Here's how the part is built. I have some questions about the finished solid (model axes, mm). Face numbers are marked on the shaded views. A direction names the side the tool comes from. Coordinates: 2 decimals unless noted, no trailing zeros. Write each loop counter-clockwise with the first axis right and the second up, starting at its lowest first coordinate (ties: lowest second). Pieces come first, ordered by that corner, then holes.
Item 1: I want a section at A-A (y = 17). Please give me the cut outline in (x, z), and give its area (3 significant figures).
Item 2: I'm going to push flat-ended pins straight in: P1, Ø2.5, axis at x = 20, z = 0, coming from the +Y side; P2, Ø3.5, axis at x = 0, z = 20, coming from the +Y side; P3, Ø1.5, axis at y = 6.5, z = 4.5, coming from the -X side; P4, Ø10, axis at x = 20, z = -7.5, coming from the -Y side. Where does each tip first touch, or does it pass through?
Item 3: Please list where these lines run through material, in increasing order: line 1 (X direction, y = 18.1, z = 0); line 2 (Z direction, x = 1, y = 17); line 3 (Z direction, x = 2, y = 3).
Item 4: For the marked faces 4, 5 and 6, which set-ups out of +Z, -Z, +X, -X, +Y, -Y let a thin tool reach every point of the face, with its end or its side?
Item 5: If we mould it in two halves opening along Z, with no side actions, what happens to the marked faces 1, 2 and 3? For each: pulls with the +Z half, pulls with the -Z half, needs draft (parallel to the pull), parting line crosses it, or undercut.
Item 6: I want a section at C-C (z = 20). Please give me the cut outline in (x, y).
Item 7: I want a section at D-D (y = 11). Please give me the cut outline in (x, z).
Item 8: I want a section at B-B (x = 20). Please give me the cut outline in (y, z).
from build123d import *

# Parameters (mm, degrees)
SKETCH1_R           = 17.5
BOSS_EXTRUDE1_DEPTH = 16
SKETCH2_R           = 25
SKETCH2_R_2         = 12.5
BOSS_EXTRUDE2_DEPTH = 4
SKETCH3_R           = 1.5
CUT_EXTRUDE1_DEPTH  = 41.620192023
CHAMFER1_SIZE       = 1
SKETCH4_R           = 12.5
BOSS_EXTRUDE3_DEPTH = 4


with BuildPart() as part:
    # Sketch1 → Boss-Extrude1 (new body)
    with BuildSketch(Plane(origin=(0, 0, 0), x_dir=(1, 0, 0), z_dir=(0, 1, 0))):
        with Locations(Location((0, 0, 0), (0, 0, 270))):
            Circle(SKETCH1_R)
        Polygon((5.773502692, -10), (11.547005384, 0), (5.773502692, 10), (-5.773502692, 10), (-11.547005384, 0), (-5.773502692, -10), align=None, mode=Mode.SUBTRACT)
    extrude(amount=BOSS_EXTRUDE1_DEPTH)

    # Sketch2 → Boss-Extrude2 (add)
    with BuildSketch(Plane(origin=(0, 16, 0), x_dir=(1, 0, 0), z_dir=(0, 1, 0))):
        with Locations(Location((0, 0, 0), (0, 0, 270))):
            Circle(SKETCH2_R)
        with Locations(Location((0, 0, 0), (0, 0, 270))):
            Circle(SKETCH2_R_2, mode=Mode.SUBTRACT)
    extrude(amount=BOSS_EXTRUDE2_DEPTH)

    # Sketch3 → Cut-Extrude1 (cut, through all)
    with BuildSketch(Plane(origin=(0, 20, 0), x_dir=(1, 0, 0), z_dir=(0, 1, 0))):
        with Locations(Location((0, 20, 0), (0, 0, 270))):
            Circle(SKETCH3_R)
        with Locations(Location((20, 0, 0), (0, 0, 270))):
            Circle(SKETCH3_R)
        with Locations(Location((0, -20, 0), (0, 0, 270))):
            Circle(SKETCH3_R)
        with Locations(Location((-20, 0, 0), (0, 0, 270))):
            Circle(SKETCH3_R)
    extrude(amount=-CUT_EXTRUDE1_DEPTH, mode=Mode.SUBTRACT)

    # Chamfer1
    chamfer1_edges = [part.edges().sort_by_distance(p)[0] for p in [
        (0, 20, -21.5),
        (20, 20, -1.5),
        (0, 20, 18.5),
        (-20, 20, -1.5),
    ]]
    chamfer(chamfer1_edges, length=CHAMFER1_SIZE)

    # Sketch4 → Boss-Extrude3 (add)
    with BuildSketch(Plane(origin=(0, 16, 0), x_dir=(1, 0, 0), z_dir=(0, 1, 0))):
        Circle(SKETCH4_R)
        Polygon((-5.773502692, -10), (5.773502692, -10), (11.547005384, 0), (5.773502692, 10), (-5.773502692, 10), (-11.547005384, 0), align=None, mode=Mode.SUBTRACT)
    extrude(amount=BOSS_EXTRUDE3_DEPTH)


solid = part.part
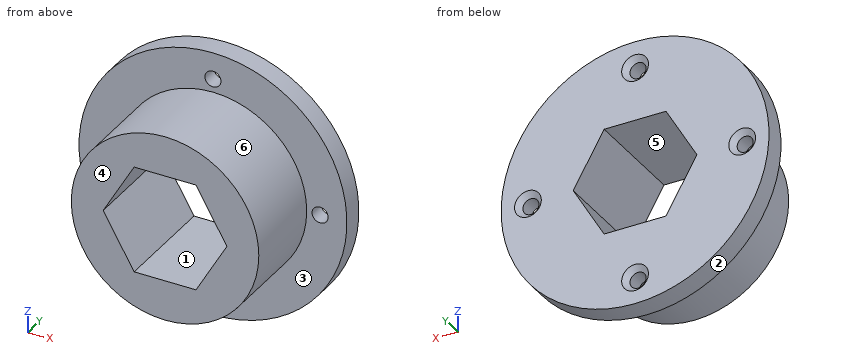
Answer:
1. outline: circle Ø50 at (0, 0); hole circle Ø3 at (-20, 0); hole (-11.55, 0) - (-5.77, -10) - (5.77, -10) - (11.55, 0) - (5.77, 10) - (-5.77, 10) - close; hole circle Ø3 at (0, -20); hole circle Ø3 at (0, 20); hole circle Ø3 at (20, 0)
1. area: 1,590 mm2
2. P1: passes through
2. P2: stops at y = 19.25
2. P3: stops at x = -17.09
2. P4: stops at y = 0
3. line 1: x = -25 to -21.5, -18.5 to -11.55, 11.55 to 18.5, 21.5 to 25
3. line 2: z = -24.98 to -21.12, -18.88 to -10, 10 to 18.88, 21.12 to 24.98
3. line 3: z = -17.39 to -10, 10 to 17.39
4. face 4: +Z, -Z, +X, -X, -Y
4. face 5: +Y, -Y
4. face 6: -Y
5. face 1: undercut
5. face 2: parting line crosses it
5. face 3: needs draft
6. outline: (-15, 16) - (-1.5, 16) - (-1.5, 19) - (-2.5, 20) - (-15, 20) - close; (1.5, 16) - (15, 16) - (15, 20) - (2.5, 20) - (1.5, 19) - close
7. outline: circle Ø35 at (0, 0); hole (-11.55, 0) - (-5.77, -10) - (5.77, -10) - (11.55, 0) - (5.77, 10) - (-5.77, 10) - close
8. outline: (16, -15) - (20, -15) - (20, -2.5) - (19, -1.5) - (16, -1.5) - close; (16, 1.5) - (19, 1.5) - (20, 2.5) - (20, 15) - (16, 15) - close
